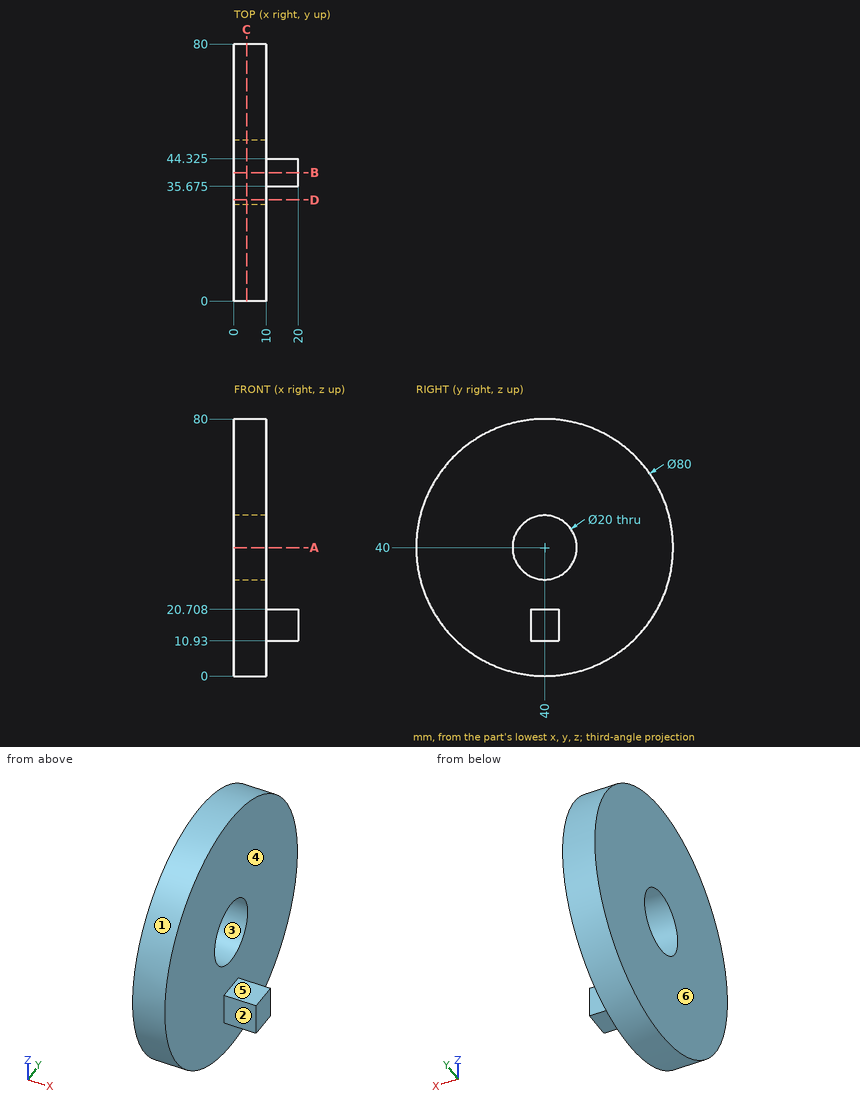
The figure shows three views and two pictorial views of one solid part (mm, origin at its lowest corner). Answer the questions. A direction names the side the tool comes from. Round coordinates to 2 decimals unless told otherwise and drop trailing zeros. Loops run counter-clockwise (first coordinate to the right, second up) from the corner with the lowest first, then second, coordinate; pieces in that order, holes last. Notation, with made-up numbers: (36.5, -7.5) - (61.5, -7.5) arc R28 ccw to (61.5, 28.5) - close; hole circle Ø2 at (51.5, -17.75). An arc over 180 degrees is marked (long way). One line per question, with ' | ' between items. Start each with the question number.
Q1. For a pull along Y with two mould halves and no side action, classify the marked faces 1, 2, 3 and 4 as +Y half, -Y half, draft (parallel to the pull), parting line (faces both ways), or undercut.
Q2. Find the intervals of material crossed by L1, parallel to Y at x = 3.25, z = 40; L2, parallel to X at y = 6.5, z = 23; L3, parallel to Y at x = 14, z = 15 (1 decimal), in increasing order.
Q3. Section B-B on y = 40 is taken. Give the vertices of the cut face in (x, z).
Q4. Section C-C on x = 4 is taken. Give the vertices of the cut face in (y, z).
Q5. Section A-A on z = 40 is taken. Give the vertices of the cut face in (x, y).
Q6. Flat-ended cylindrical pins translate along their axes: pin 1 (4.5 mm diameter, centred on x = 17, y = 42, fed in from -Z); pin 2 (12 mm diameter, centred on x = 8, y = 17.5, fed in from -Z); pin 3 (12 mm diameter, centred on x = 9.5, z = 13, fed in from +Y) (1 decimal); pin 4 (18 mm diameter, centred on y = 40, z = 40, fed in from -X). Find the tip coordinate at first contact, or state that the pin passes through.
Q7. For the marked faces 5 and 6, determine the directions among +Z, -Z, +X, -X, +Y, -Y from which every point of the face is accessible in a straight line to the end or side of a thin tool.
Q8. Section D-D on y = 31.5 is taken. Give the vertices of the cut face in (x, z).
Established:
1) face 1: parting line | face 2: -Y half | face 3: undercut | face 4: draft
2) L1: 0 to 30, 50 to 80 | L2: 0 to 10 | L3: 35.7 to 44.3
3) outline: (0, 0) - (10, 0) - (10, 10.93) - (20, 10.93) - (20, 20.71) - (10, 20.71) - (10, 30) - (0, 30) - close; (0, 50) - (10, 50) - (10, 80) - (0, 80) - close
4) outline: circle Ø80 at (40, 40); hole circle Ø20 at (40, 40)
5) outline: (0, 0) - (10, 0) - (10, 30) - (0, 30) - close; (0, 50) - (10, 50) - (10, 80) - (0, 80) - close
6) pin 1: z = 10.93 | pin 2: z = 3.56 | pin 3: y = 74 | pin 4: through
7) face 5: +Z, +X, +Y, -Y | face 6: +Z, -Z, -X, +Y, -Y
8) outline: (0, 0.91) - (10, 0.91) - (10, 34.73) - (0, 34.73) - close; (0, 45.27) - (10, 45.27) - (10, 79.09) - (0, 79.09) - close
